from build123d import *

# Parameters (mm, degrees)
F0_W     = 70
F0_H     = 70
F0_R     = 5.0038
F0_R_2   = 12.7
F0_R_3   = 5
F1_DEPTH = 6
F2_R     = 3
F3_W     = 44.45
F3_H     = 44.45
F3_W_2   = 38.1
F3_H_2   = 38.1
F4_DEPTH = 15


with BuildPart() as f1:
    # F0 (on Top) → F1 (new body)
    with BuildSketch(Plane.XY):
        Rectangle(F0_W, F0_H)
        with Locations((-27.4562, -27.4562)):
            Circle(F0_R, mode=Mode.SUBTRACT)
        with Locations((27.4562, -27.4562)):
            Circle(F0_R, mode=Mode.SUBTRACT)
        with Locations((-27.4562, 27.4562)):
            Circle(F0_R, mode=Mode.SUBTRACT)
        Circle(F0_R_2, mode=Mode.SUBTRACT)
        with Locations((27.46, 27.46)):
            Circle(F0_R_3, mode=Mode.SUBTRACT)
    extrude(amount=F1_DEPTH)

    # F2
    f2_edges = [f1.edges().sort_by_distance(p)[0] for p in [
        (-12.7, 0, 0),
    ]]
    fillet(f2_edges, radius=F2_R)

    # F3 (on face) → F4 (join)
    with BuildSketch(Plane.XY.offset(6)):
        Rectangle(F3_W, F3_H)
        Rectangle(F3_W_2, F3_H_2, mode=Mode.SUBTRACT)
    extrude(amount=F4_DEPTH)


solid = f1.part
Input: part model. Units: mm. Frame: model coordinates. A direction names the side the tool comes from. Coordinates: 2 decimals unless noted, no trailing zeros. Loops run counter-clockwise (first coordinate to the right, second up) from the corner with the lowest first, then second, coordinate; pieces in that order, holes last.
Q1. Set-up query: faces 4 (the face through (19.05, 0, 13)), 5 (the face through (0, 22.225, 13)), 6 (the face through (0, -22.225, 13)). Return all of +Z, -Z, +X, -X, +Y, -Y with unobstructed straight access to the full face (end or side cutting, diameter ignored); none if empty.
Q2. Draft query along Y for faces 1 (the face through (0, 19.05, 13)), 2 (the face through (0, -35, 3)), 3 (the face through (0, 35, 3)). Return one class per face: +Y half, -Y half, draft (parallel to the pull), parting line (faces both ways), or undercut.
Q3. Cut plane A-A (x = 0). Output: boundary loops of the cut face in (y, z) (3 decimals).
Q4. Material intervals for line 1 (X direction, y = -5, z = 15.5) (3 decimals); line 2 (Y direction, x = -28, z = 4), sorted ascending.
Q5. Cut plane C-C (x = 27.46). Output: boundary loops of the cut face in (y, z), then the cut area to 3 significant figures.
Q6. Contact query for flat-ended pins moving along their axis: pin 1 (6 mm diameter, centred on x = 27.46, y = 27.46, fed in from -Z); pin 2 (4.5 mm diameter, centred on y = -5, z = 15, fed in from -X) (3 decimals); pin 3 (4.5 mm diameter, centred on x = -9, z = 10.5, fed in from -Y) (3 decimals); pin 4 (1.5 mm diameter, centred on x = 25.5, y = 19, fed in from +Z). Output: stop coordinate, or through.
Q7. Cut plane B-B (z = 14.5). Output: boundary loops of the cut face in (x, y) (3 decimals), then the cut area to 3 significant figures.
Working result:
1. face 4: +Z
1. face 5: +Z, +X, -X, +Y
1. face 6: +Z, +X, -X, -Y
2. face 1: undercut
2. face 2: -Y half
2. face 3: +Y half
3. outline: (-35, 0) - (-15.7, 0) arc R3 ccw to (-12.7, 3) - (-12.7, 6) - (-19.05, 6) - (-19.05, 21) - (-22.225, 21) - (-22.225, 6) - (-35, 6) - close; (12.7, 3) arc R3 ccw to (15.7, 0) - (35, 0) - (35, 6) - (22.225, 6) - (22.225, 21) - (19.05, 21) - (19.05, 6) - (12.7, 6) - close
4. line 1: x = -22.225 to -19.05, 19.05 to 22.225
4. line 2: y = -35 to -32.43, -22.48 to 22.48, 32.43 to 35
5. outline: (-35, 0) - (-32.46, 0) - (-32.46, 6) - (-35, 6) - close; (-22.45, 0) - (22.46, 0) - (22.46, 6) - (-22.45, 6) - close; (32.46, 0) - (35, 0) - (35, 6) - (32.46, 6) - close
5. area: 300 mm2
6. pin 1: passes through
6. pin 2: stops at x = -22.225
6. pin 3: stops at y = -22.225
6. pin 4: stops at z = 6
7. outline: (-22.225, -22.225) - (22.225, -22.225) - (22.225, 22.225) - (-22.225, 22.225) - close; hole (-19.05, -19.05) - (19.05, -19.05) - (19.05, 19.05) - (-19.05, 19.05) - close
7. area: 524 mm2
